```python
from build123d import *

# Parameters (mm, degrees)
SKETCH1_W               = 175
SKETCH1_H               = 175
BOSS_EXTRUDE1_DEPTH     = 5
SKETCH2_R               = 2
CUT_EXTRUDE1_DEPTH      = 5
SKETCH3_W               = 160
SKETCH3_H               = 6
SKETCH3_W_2             = 145
BOSS_EXTRUDE3_DEPTH     = 18
SKETCH4_R               = 2
CUT_EXTRUDE2_DEPTH      = 1
CUT_EXTRUDE2_DEPTH_BACK = 176
SKETCH5_R               = 5
CUT_EXTRUDE3_DEPTH      = 2.5


with BuildPart() as part:
    # Sketch1 → Boss-Extrude1 (new body)
    with BuildSketch(Plane(origin=(0, 0, 0), x_dir=(1, 0, 0), z_dir=(0, 1, 0))):
        with Locations((-24.045801527, -27.385496183)):
            Rectangle(SKETCH1_W, SKETCH1_H)
    extrude(amount=BOSS_EXTRUDE1_DEPTH)

    # Sketch2 → Cut-Extrude1 (cut)
    with BuildSketch(Plane(origin=(0, 5, 0), x_dir=(1, 0, 0), z_dir=(0, 1, 0))):
        with Locations((-106.545801527, 55.114503817)):
            Circle(SKETCH2_R)
        with Locations((53.454198473, 55.114503817)):
            Circle(SKETCH2_R)
        with Locations((53.454198473, -99.885496183)):
            Circle(SKETCH2_R)
        with Locations((-106.545801527, -78.885496183)):
            Circle(SKETCH2_R)
    extrude(amount=-CUT_EXTRUDE1_DEPTH, mode=Mode.SUBTRACT)

    # Sketch3 → Boss-Extrude3 (add)
    with BuildSketch(Plane.XZ):
        with Locations((-31.545801527, 111.885496183)):
            Rectangle(SKETCH3_W, SKETCH3_H)
        with Locations((-24.045801527, -57.114503817)):
            Rectangle(SKETCH3_W_2, SKETCH3_H)
    extrude(amount=BOSS_EXTRUDE3_DEPTH)

    # Sketch4 → Cut-Extrude2 (cut, two sides)
    with BuildSketch(Plane(origin=(0, 0, -60.114503817), x_dir=(-1, 0, 0), z_dir=(0, 0, -1))) as cut_extrude2_sk:
        with Locations((-28.454198473, -8.900832872)):
            Circle(SKETCH4_R)
        with Locations((24.045801527, -8.900832872)):
            Circle(SKETCH4_R)
        with Locations((76.545801527, -8.900832872)):
            Circle(SKETCH4_R)
    extrude(amount=CUT_EXTRUDE2_DEPTH, mode=Mode.SUBTRACT)
    extrude(cut_extrude2_sk.sketch, amount=-CUT_EXTRUDE2_DEPTH_BACK, mode=Mode.SUBTRACT)

    # Sketch5 → Cut-Extrude3 (cut)
    with BuildSketch(Plane(origin=(0, 0, -60.114503817), x_dir=(-1, 0, 0), z_dir=(0, 0, -1))):
        with Locations((-28.454198473, -8.900832872)):
            Circle(SKETCH5_R)
        with Locations((24.045801527, -8.900832872)):
            Circle(SKETCH5_R)
        with Locations((76.545801527, -8.900832872)):
            Circle(SKETCH5_R)
    extrude(amount=-CUT_EXTRUDE3_DEPTH, mode=Mode.SUBTRACT)


solid = part.part
```
CAD build for the part. Positions are in the model's coordinates, mm. A direction names the side the tool comes from. Round coordinates to 2 decimals unless told otherwise and drop trailing zeros. Loops run counter-clockwise (first coordinate to the right, second up) from the corner with the lowest first, then second, coordinate; pieces in that order, holes last. Notation, with made-up numbers: (28, -34.75) - (53, -34.75) arc R23 ccw to (53, -2.75) - close; hole circle Ø7 at (71.25, 43). An arc over 180 degrees is marked (long way). Return JSON: item names as keys, results as strings. Group by question number.
Q1. Band-saw the part on B-B on z = 40. Give the cut face in (x, y).
Q2. Two-plate mould, pull along Z, no slides. Class faces 5 (the face through (-33, -9, 108.885)), 6 (the face through (26, -9, -57.615)), 7 (the face through (-74.548, -8.813, -55.889)): +Z half, -Z half, draft (parallel to the pull), parting line (faces both ways), or undercut.
Q3. Flat gauge pins, fed straight in: pin 1 Ø10 at (x, z) = (-15, 71.5) entering from -Y; pin 2 Ø6.5 at (y, z) = (-8, 113) entering from +X; pin 3 Ø3 at (x, y) = (-24.05, -8.9) entering from -Z. Where does each tip first touch, or does it go through?
Q4. Drill centre lines: line 1 along Z through (x, y) = (-64, -6); line 2 along Y through (x, z) = (-34.5, -9); line 3 along Z through (x, y) = (28, -12.25). Where is each one in solid material? Low to high. Write a range as [from, to].
Q5. Band-saw the part on A-A on x = -5. Give the cut face in (y, z).
Q6. Tool access for faces 1 (the face through (-96.546, -9, -57)), 2 (the face through (-74.548, -8.813, 111.843)), 3 (the face through (48.454, -9, -57)), 4 (the face through (-71.55, -8.68, -58.88)): list every direction of +Z, -Z, +X, -X, +Y, -Y with a clear straight run to the whole face (end or side of a thin tool).
Q7. Band-saw the part on C-C on x = -100. Give the cut face in (y, z).
Solutions:
{
 "1": {"outline": "(-111.55, 0) - (63.45, 0) - (63.45, 5) - (-111.55, 5) - close"},
 "2": {"face 5": "undercut", "face 6": "-Z half", "face 7": "draft"},
 "3": {"pin 1": "stops at y = 0", "pin 2": "stops at x = 48.45", "pin 3": "passes through"},
 "4": {"line 1": "z = [-60.11, -54.11], [108.89, 114.89]", "line 2": "y = [0, 5]", "line 3": "z = [-57.61, -54.11], [108.89, 114.89]"},
 "5": {"outline": "(-18, -60.11) - (5, -60.11) - (5, 114.89) - (-18, 114.89) - (-18, 108.89) - (0, 108.89) - (0, -54.11) - (-18, -54.11) - close"},
 "6": {"face 1": "-Z, -X, -Y", "face 2": "+Z, -Z", "face 3": "+Z, -Z, +X, -Y", "face 4": "-Z"},
 "7": {"outline": "(-18, 108.89) - (0, 108.89) - (0, -60.11) - (5, -60.11) - (5, 114.89) - (-18, 114.89) - close"}
}
